For this review, take the finished solid that the model builds, in its own axes (mm). A direction names the side the tool comes from. Coordinates: 2 decimals unless noted, no trailing zeros. Loops run counter-clockwise (first coordinate to the right, second up) from the corner with the lowest first, then second, coordinate; pieces in that order, holes last. Notation, with made-up numbers: M 23,82.5 L 76,82.5 A15 ccw 76,94.5 Z; hole C -5.5,52 d4. An arc over 180 degrees is marked long. Write each question's results on one line, items separated by ' | '. Start each with the question number.
```python
from build123d import *

# Parameters (mm, degrees)
CROQUIS1_R              = 1.5
SALIENTE_EXTRUIR1_DEPTH = 5


with BuildPart() as part:
    # Croquis1 → Saliente-Extruir1 (new body)
    with BuildSketch(Plane.XY):
        with BuildLine():
            Line((-28.790532902, 40.226856436), (-28.790532902, 20.926856436))
            Line((-28.790532902, 20.926856436), (-28.790532902, -0.073143564))
            Line((-28.790532902, -0.073143564), (-28.790532902, -3.773143564))
            ThreePointArc((-28.790532902, -3.773143564), (-26.740280371, -8.722891033), (-21.790532902, -10.773143564))
            Line((-21.790532902, -10.773143564), (-1.440532902, -10.773143564))
            ThreePointArc((-1.440532902, -10.773143564), (2.386301421, -10.011938889), (5.630534909, -7.844211376))
            Line((5.630534909, -7.844211376), (5.630534909, 17.997924248))
            ThreePointArc((5.630534909, 17.997924248), (2.386301421, 20.165651761), (-1.440532902, 20.926856436))
            Line((-1.440532902, 20.926856436), (-13.790532902, 20.926856436))
            ThreePointArc((-13.790532902, 20.926856436), (-18.740280371, 22.977108967), (-20.790532902, 27.926856436))
            Line((-20.790532902, 27.926856436), (-20.790532902, 40.226856436))
            Line((-20.790532902, 40.226856436), (-28.790532902, 40.226856436))
        make_face()
        with Locations((-25.790532902, -4.773143564)):
            Circle(CROQUIS1_R, mode=Mode.SUBTRACT)
        with Locations((-25.790532902, 5.226856436)):
            Circle(CROQUIS1_R, mode=Mode.SUBTRACT)
        with Locations((-15.290532902, 5.076856436)):
            Circle(CROQUIS1_R, mode=Mode.SUBTRACT)
        with Locations((-7.290532902, -4.423143564)):
            Circle(CROQUIS1_R, mode=Mode.SUBTRACT)
        with Locations((-7.290532902, 5.076856436)):
            Circle(CROQUIS1_R, mode=Mode.SUBTRACT)
        with Locations((-7.290532902, 14.576856436)):
            Circle(CROQUIS1_R, mode=Mode.SUBTRACT)
        with Locations((0.709467098, 5.076856436)):
            Circle(CROQUIS1_R, mode=Mode.SUBTRACT)
        with Locations((-25.790532902, 25.226856436)):
            Circle(CROQUIS1_R, mode=Mode.SUBTRACT)
        with Locations((-25.790532902, 35.226856436)):
            Circle(CROQUIS1_R, mode=Mode.SUBTRACT)
    extrude(amount=SALIENTE_EXTRUIR1_DEPTH)


solid = part.part
```
Q1. Take a section at B-B, the plane x = -25. Give the boundary of the cut face in (y, z), then the cut area to 3 significant figures.
Q2. The part is to be moulded in two halves that separate along X. For faces 1 (the face through (-26.79, -8.67, 2.46)), 2 (the face through (-18.686, 22.923, 2.465)), 3 (the face through (-16.79, 5.14, 2.46)), 4 (the face through (-26.896, 36.241, 2.465)), say which applies: pulls with the +X half, pulls with the -X half, needs draft (parallel to the pull), parting line crosses it, or undercut.
Q3. Insertion check: P1, Ø1, axis at x = -16, z = 3.5, coming from the +Y side. The pin has a flat end and moves straight along its axis. Give the tip position at first contact, or say it passes through.
Q4. Take a section at D-D, the plane y = 19.5. Give the boundary of the cut face in (x, z), then the cut area to 3 significant figures.
Q5. Take a section at C-C, the plane z = 2.85. Give the number of separate pieces and of enclosed holes in the cut face, then the cut area to 3 significant figures.
Q6. For faces 5 (the face through (-12, 9, 0)), 6 (the face through (-20.791, 34, 2)), list the 3-axis set-ups (+Z, -Z, +X, -X, +Y, -Y) from which the entire face can be reached by the end or side of a thin tool; tool diameter is ignored.
Q7. Take a section at A-A, the plane x = -16. Give the boundary of the cut face in (y, z), then the cut area to 3 significant figures.
Q8. To check wall thickness, follow line 1 along Y through (x, z) = (-24.5, 4); line 2 along X through (y, z) = (32.5, 3.75); line 3 along Y through (x, z) = (-4.5, 3.65). State the ranges of each line that lie inside material, in increasing order.
Results:
1) outline: M -9.99,0 L -6.05,0 L -6.05,5 L -9.99,5 Z; M -3.5,0 L 3.95,0 L 3.95,5 L -3.5,5 Z; M 6.5,0 L 23.95,0 L 23.95,5 L 6.5,5 Z; M 26.5,0 L 33.95,0 L 33.95,5 L 26.5,5 Z; M 36.5,0 L 40.23,0 L 40.23,5 L 36.5,5 Z | area: 200 mm^2
2) face 1: pulls with the -X half | face 2: pulls with the +X half | face 3: undercut | face 4: undercut
3) P1: y = 21.47
4) outline: M -28.79,0 L 3.71,0 L 3.71,5 L -28.79,5 Z | area: 162 mm^2
5) separate pieces: 1 | enclosed holes: 9 | area: 1,170 mm^2
6) face 5: -Z, +X, -X, +Y, -Y | face 6: +Z, -Z, +X, +Y
7) outline: M -10.77,0 L 3.76,0 L 3.76,5 L -10.77,5 Z; M 6.4,0 L 21.28,0 L 21.28,5 L 6.4,5 Z | area: 147 mm^2
8) line 1: -10.23 to -5.54, -4.01 to 4.46, 5.99 to 24.46, 25.99 to 34.46, 35.99 to 40.23 | line 2: -28.79 to -20.79 | line 3: -10.77 to 20.93
